```python
from build123d import *

# Parameters (mm, degrees)
BOSS_EXTRUDE1_DEPTH     = 198.6
CUT_EXTRUDE1_DEPTH      = 1
CUT_EXTRUDE1_DEPTH_BACK = 199.6


with BuildPart() as part:
    # Sketch4 → Boss-Extrude1 (new body)
    with BuildSketch(Plane.XY):
        with BuildLine():
            Line((0, -5.45), (0.655464476, -6))
            Line((0.655464476, -6), (4.504469158, -6))
            Line((4.504469158, -6), (8.25, -9.745530842))
            Line((8.25, -9.745530842), (8.25, -12.885))
            Line((8.25, -12.885), (4, -12.885))
            Line((4, -12.885), (4, -14.45))
            Line((4, -14.45), (4.55, -14.45))
            Line((4.55, -14.45), (4.55, -15))
            Line((4.55, -15), (12.885, -15))
            ThreePointArc((12.885, -15), (14.380530842, -14.380530842), (15, -12.885))
            Line((15, -12.885), (15, -4.55))
            Line((15, -4.55), (14.45, -4.55))
            Line((14.45, -4.55), (14.45, -4))
            Line((14.45, -4), (12.885, -4))
            Line((12.885, -4), (12.885, -8.25))
            Line((12.885, -8.25), (9.745530842, -8.25))
            Line((9.745530842, -8.25), (6, -4.504469158))
            Line((6, -4.504469158), (6, -0.655464476))
            Line((6, -0.655464476), (5.45, 0))
            Line((5.45, 0), (3.5, 0))
            ThreePointArc((3.5, 0), (3.371433308, -0.939913534), (2.995178599, -1.81077474))
            Line((2.995178599, -1.81077474), (4.675743591, -3.491339732))
            Line((4.675743591, -3.491339732), (3.491339732, -4.675743591))
            Line((3.491339732, -4.675743591), (1.81077474, -2.995178599))
            ThreePointArc((1.81077474, -2.995178599), (0.939913534, -3.371433308), (0, -3.5))
            Line((0, -3.5), (0, -5.45))
        make_face()
        with BuildLine():
            Line((9.375, -10.365), (9.375, -12.885))
            ThreePointArc((9.375, -12.885), (9.664964287, -13.585035713), (10.365, -13.875))
            Line((10.365, -13.875), (12.885, -13.875))
            ThreePointArc((12.885, -13.875), (13.585035713, -13.585035713), (13.875, -12.885))
            Line((13.875, -12.885), (13.875, -10.365))
            ThreePointArc((13.875, -10.365), (13.585035713, -9.664964287), (12.885, -9.375))
            Line((12.885, -9.375), (10.365, -9.375))
            ThreePointArc((10.365, -9.375), (9.664964287, -9.664964287), (9.375, -10.365))
        make_face(mode=Mode.SUBTRACT)
    extrude(amount=BOSS_EXTRUDE1_DEPTH)

    # Mirror1: part across plane


with BuildPart() as part_1:
    add(part.part)
    add(part.part.mirror(Plane(origin=(0, 0, 0), x_dir=(0, 0, 1), z_dir=(1, 0, 0))))

    # Mirror2: part across plane


with BuildPart() as part_2:
    add(part_1.part)
    add(part_1.part.mirror(Plane.ZX))

    # Sketch5 → Cut-Extrude1 (cut, two sides)
    with BuildSketch(Plane.XY.offset(198.6)) as cut_extrude1_sk:
        Polygon((-5.675, 12.885), (-5.4, 13.16), (-5.125, 12.885), align=None)
    extrude(amount=CUT_EXTRUDE1_DEPTH, mode=Mode.SUBTRACT)
    extrude(cut_extrude1_sk.sketch, amount=-CUT_EXTRUDE1_DEPTH_BACK, mode=Mode.SUBTRACT)


solid = part_2.part
```
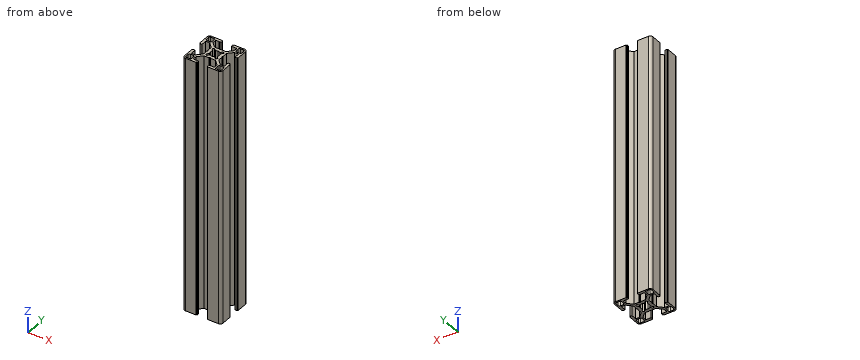
Model file for the job. Use its own axes, mm. Coordinates: 2 decimals unless noted, no trailing zeros. Return JSON: item names as keys, results as strings.
Item 1: Wall check: line 1 along Y through (x, z) = (9.5, 94); line 2 along X through (y, z) = (-9.75, 34); line 3 along Y through (x, z) = (-13, 133). Give the ranges that are in metal, low to high. Write a range as from..to.
Model answer:
{"line 1": "y = -15..-13.37, -9.88..-8, 8..9.88, 13.37..15", "line 2": "x = -15..-13.66, -9.59..-8.25, 8.25..9.59, 13.66..15", "line 3": "y = -15..-13.87, -9.38..-4, 4..9.38, 13.87..15"}
Item 2: Pin check, flat tips, straight feed: P1, Ø1.5, axis at x = 2.5, y = 2.5, coming from the +Z side; P2, Ø0.8, axis at y = 13.5, z = 106, coming from the +X side; P3, Ø0.6, axis at x = -14.5, z = 91, coming from the +Y side; P4, Ø3, axis at x = 3, z = 66.5, coming from the +Y side. Stop position of each tip, or through.
Model answer:
{"P1": "passes through", "P2": "stops at x = 14.99", "P3": "stops at y = 14.54", "P4": "stops at y = 14.45"}
Item 3: Slice it at A-A (z = 73.5). Count the separate pieces of the cut face and the enclosed holes in it, then the cut area to 3 significant figures.
Model answer:
{"separate pieces": "1", "enclosed holes": "5", "area": "295 mm²"}
